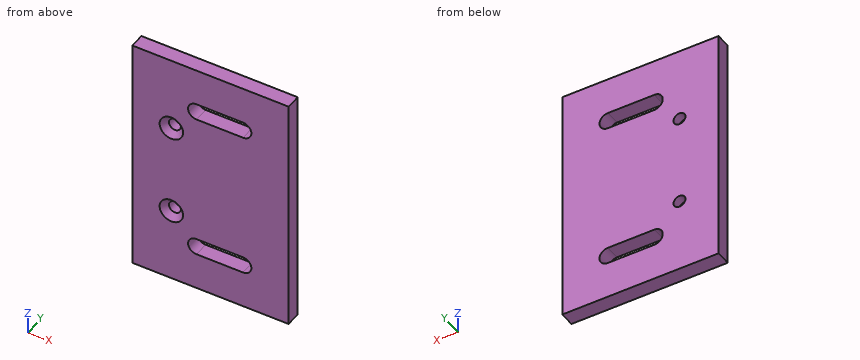
Autodesk Inventor part; units mm, degrees
ref_plane "YZ Plane" through (0, 0, 0) normal (1, 0, 0) x (0, 1, 0)
ref_plane "XZ Plane" through (0, 0, 0) normal (0, 1, 0) x (-1, 0, 0)
ref_plane "XY Plane" through (0, 0, 0) normal (0, 0, 1) x (1, 0, 0)
sketch "Sketch1" plane through (0, 0, 0) normal (0, 1, 0) x (-1, 0, 0)
  arc A0 (23.5, 20) -> (23.5, 29) centre (23.5, 24.5) ccw
  line L0 (23.5, 20) -> (-1.5, 20)
  line L1 (23.5, 29) -> (-1.5, 29)
  arc A1 (-1.5, 29) -> (-1.5, 20) centre (-1.5, 24.5) ccw
  arc A2 (23.5, 100) -> (23.5, 109) centre (23.5, 104.5) ccw
  line L2 (23.5, 100) -> (-1.5, 100)
  line L3 (23.5, 109) -> (-1.5, 109)
  arc A3 (-1.5, 109) -> (-1.5, 100) centre (-1.5, 104.5) ccw
  line L4 (74, 129) -> (0, 129)
  line L5 (0, 129) -> (74, 129)
  line L6 (74, 129) -> (74, 0)
  line L7 (74, 0) -> (0, 0)
  line L8 (0, 0) -> (0, 129)
  line L9 (0, 129) -> (-26, 129)
  line L10 (-26, 129) -> (-26, 0)
  line L11 (-26, 0) -> (0, 0)
  line L12 (0, 0) -> (0, 129)
  line L13 (74, 0) -> (58, 0)
  line L14 (58, 0) -> (58, 129)
  line L15 (58, 129) -> (74, 129)
  line L16 (74, 129) -> (74, 0)
  point P0 (0, 0)
  point P1 (23.5, 104.5)
  point P2 (0, 109)
  point P3 (0, 20)
  point P4 (0, 29)
  point P5 (0, 100)
  dimension "d98" = 74
  dimension "d106" = 26
  dimension "d118" = 16
extrude "Extrusion1" add sketch "Sketch1" along normal blind 8 contours A0 L1 L8 L2 A2 L3 L4 L14 L7 L0 | L8 L11 L10 L9 L3 A3 L2 L1 A1 L0
sketch "Sketch4" plane through (0, 0, 0) normal (0, -1, 0) x (1, 0, 0)
  line L0 (-74, 0) -> (-74, 129)
  line L1 (-74, 129) -> (0, 0)
  line L2 (0, 100) -> (0, 0)
  line L3 (0, 129) -> (-74, 0)
  line L4 (-37, 0) -> (-37, 129)
  line L5 (-58, 129) -> (26, 129)
  line L6 (-37, 129) -> (-37, 89)
  line L7 (-37, 129) -> (3, 129) construction
  line L8 (-37, 89) -> (-37, 40)
  line L9 (-37, 40) -> (-37, 0)
  point P0 (-37, 64.5)
  dimension "d119" = 40
  dimension "d120" = 90
  dimension "d121" = 49
  dimension "d122" = 40
hole "Hole1" at (-37, 0, 89) at (-37, 0, 40) direction (0, 1, 0) diameter 6.4 depth 20 countersink diameter 12.6 countersink angle 90
properties part number "Halterung_Führungsschiene_Version2"
Verification items for the finished model (mm, model axes). Round coordinates to 2 decimals unless told otherwise and drop trailing zeros. Write each loop counter-clockwise with the first axis right and the second up, starting at its lowest first coordinate (ties: lowest second). Pieces come first, ordered by that corner, then holes.
1. Gauge pin test, flat ends, axial feed: P1, Ø4, axis at x = -37, z = 40, coming from the +Y side; P2, Ø12, axis at x = 8.5, z = 47.5, coming from the -Y side; P3, Ø7.5, axis at x = -37, z = 89, coming from the -Y side. Record the tip position at first contact, or that the pin passes through.
2. Section check D-D on x = -37. Enter the section's corners in (y, z).
3. Section check C-C on y = 5.5. Enter the section's corners in (x, z), plus the area to 3 significant figures.
4. Section check A-A on x = -21. Enter the section's corners in (y, z).
5. Scan lines: L1, parallel to Z at x = -7.5, y = 4.25; L2, parallel to X at y = 4.65, z = 40; L3, parallel to Z at x = -38, y = 1.5. Record each from-to range of solid material in increasing order.
6. Section check B-B on z = 89. Enter the section's corners in (x, y), plus the area to 3 significant figures.
Answer:
1. P1: passes through
1. P2: stops at y = 0
1. P3: stops at y = 2.55
2. outline: (0, 0) - (8, 0) - (8, 36.8) - (3.1, 36.8) - (0, 33.7) - close; (0, 46.3) - (3.1, 43.2) - (8, 43.2) - (8, 85.8) - (3.1, 85.8) - (0, 82.7) - close; (0, 95.3) - (3.1, 92.2) - (8, 92.2) - (8, 129) - (0, 129) - close
3. outline: (-58, 0) - (26, 0) - (26, 129) - (-58, 129) - close; hole circle Ø6.4 at (-37, 40); hole circle Ø6.4 at (-37, 89); hole (-23.5, 20) - (1.5, 20) arc R4.5 ccw to (1.5, 29) - (-23.5, 29) arc R4.5 ccw to start; hole (-23.5, 100) - (1.5, 100) arc R4.5 ccw to (1.5, 109) - (-23.5, 109) arc R4.5 ccw to start
3. area: 10,200 mm2
4. outline: (0, 0) - (8, 0) - (8, 20) - (0, 20) - close; (0, 29) - (8, 29) - (8, 100) - (0, 100) - close; (0, 109) - (8, 109) - (8, 129) - (0, 129) - close
5. L1: z = 0 to 20, 29 to 100, 109 to 129
5. L2: x = -58 to -40.2, -33.8 to 26
5. L3: z = 0 to 35.31, 44.69 to 84.31, 93.69 to 129
6. outline: (-58, 0) - (-43.3, 0) - (-40.2, 3.1) - (-40.2, 8) - (-58, 8) - close; (-33.8, 3.1) - (-30.7, 0) - (26, 0) - (26, 8) - (-33.8, 8) - close
6. area: 611 mm2
